```python
from build123d import *

# Parameters (mm, degrees)
F1_DEPTH = 10
F2_SIZE  = 2
F3_R     = 2.5
F4_DEPTH = 25
F5_DEPTH = 25


with BuildPart() as f1:
    # F0 (on Top) → F1 (new body)
    with BuildSketch(Plane.XY):
        with BuildLine():
            ThreePointArc((-2, 0), (-0.5857864376, 0.5857864376), (0, 2))
            Line((0, 2), (0, 20))
            Line((0, 20), (-3, 20))
            Line((-3, 20), (-3, 8))
            Line((-3, 8), (-3.0090067523, 8))
            ThreePointArc((-3.0090067523, 8), (-8.5090067523, 2.5), (-14.0090067523, 8))
            Line((-14.0090067523, 8), (-15, 8))
            Line((-15, 8), (-15, 2))
            ThreePointArc((-15, 2), (-14.4142135624, 0.5857864376), (-13, 0))
            Line((-13, 0), (-2, 0))
        make_face()
    extrude(amount=F1_DEPTH)

    # F2
    f2_edges = [f1.edges().sort_by_distance(p)[0] for p in [
        (-14.504503, 8, 10),
        (-14.504503, 8, 0),
        (-1.5, 20, 10),
        (-1.5, 20, 0),
    ]]
    chamfer(f2_edges, length=F2_SIZE)

    # F3 (on face) → F4 (cut)
    with BuildSketch(Plane(origin=(-3, 0, 0), x_dir=(0, -1, 0), z_dir=(-1, 0, 0))):
        with Locations((-15, 5)):
            Circle(F3_R)
    extrude(amount=-F4_DEPTH, mode=Mode.SUBTRACT)

    # F5 (add): a face of the model
    f5_faces = [f1.faces().sort_by_distance(p)[0] for p in [
        (0, 10.2845386319, 5),
    ]]
    extrude(f5_faces, amount=F5_DEPTH)


solid = f1.part
```
The model under review builds one solid part; all positions refer to its coordinate system, in mm. A direction names the side the tool comes from. Round coordinates to 2 decimals unless told otherwise and drop trailing zeros. Order: outer loops, then holes, each group sorted by start corner. A loop starts at its lowest first (then second) coordinate and runs counter-clockwise, first axis right, second up.
Item 1: For pin 1 (3 mm diameter, centred on x = 6.5, z = 7, fed in from -Y); pin 2 (1.5 mm diameter, centred on y = 13, z = 4, fed in from +X), all flat-tipped, find the tip position at first contact; note any pin that passes through.
Working result:
pin 1: stops at y = 2
pin 2: stops at x = 25
Item 2: Draft analysis for pull direction X (two halves, no side actions). For faces 6 (the flat face through (-14.5, 7, 9)), 7 (the flat face through (-3, 11, 5)), 8 (the cylindrical face through (-8.4, 2.5, 4.9)), state which applies: released by +X, released by -X, zero draft, split by the parting line, or undercut.
Working result:
face 6: zero draft
face 7: released by -X
face 8: undercut
Item 3: Machinability: for faces 1 (the flat face through (-14.5, 7, 1)), 2 (the flat face through (12, 2, 5)), 3 (the cylindrical face through (-14.43, 0.6, 4.93)), 4 (the flat face through (-14.5, 8, 5)), 5 (the flat face through (11, 19, 1)), which of the approach directions +Z, -Z, +X, -X, +Y, -Y give a long, thin tool a straight path to every point of the face, cutting with its end or side? Answer none if there is none.
Working result:
face 1: -Z, -X, +Y
face 2: +Z, -Z, +X, -Y
face 3: +Z, -Z, -X, -Y
face 4: +Z, -Z, -X, +Y
face 5: -Z, +X, -X, +Y
Item 4: Add section C-C, the plane x = 20.5. State the section outline as (y, z) points.
Working result:
outline: (2, 0) - (18, 0) - (20, 2) - (20, 8) - (18, 10) - (2, 10) - close; hole circle Ø5 at (15, 5)
Item 5: To check wall thickness, follow probe 1 along Z at (x, y) = (8.5, 15); probe 2 along X at (y, z) = (9.5, 2.75); probe 3 along Y at (x, z) = (2, 7.75). State the ranges of each line that lie inside material, in increasing order.
Working result:
probe 1: z = 0 to 2.5, 7.5 to 10
probe 2: x = -3 to 25
probe 3: y = 2 to 20
Item 6: Add section B-B, the plane y = 15. State the section outline as (x, z) points, and give its area (3 significant figures).
Working result:
outline: (-3, 0) - (25, 0) - (25, 2.5) - (-3, 2.5) - close; (-3, 7.5) - (25, 7.5) - (25, 10) - (-3, 10) - close
area: 140 mm2
